Check sheet for the modelled part. Datum: model origin and axes. Units: mm. A direction names the side the tool comes from. Round coordinates to 2 decimals unless told otherwise and drop trailing zeros. Loops run counter-clockwise (first coordinate to the right, second up) from the corner with the lowest first, then second, coordinate; pieces in that order, holes last. Notation, with made-up numbers: (39.25, 15) -> (64.25, 15) arc R19 ccw to (64.25, 45) -> close; hole circle Ø5 at (62, -5). An arc over 180 degrees is marked (long way). One line per question, with ' | ' between items.
```python
from build123d import *

# Parameters (mm, degrees)
F0_W            = 116
F0_H            = 116
F1_DEPTH        = 20
F2_W            = 112
F2_H            = 112
F3_DEPTH        = 13
F4_W            = 96
F4_H            = 96
F5_DEPTH        = 7
F6_W            = 112
F6_H            = 112
F6_W_2          = 96
F6_H_2          = 96
F7_DEPTH        = 3.5
F8_W            = 10
F8_H            = 10
F9_DEPTH        = 7
F11_D           = 3.4
F11_CBORE_D     = 6.5
F11_CBORE_DEPTH = 3


with BuildPart() as f1:
    # F0 (on Top) → F1 (new body)
    with BuildSketch(Plane.XY):
        Rectangle(F0_W, F0_H)
    extrude(amount=F1_DEPTH)

    # F2 (on face) → F3 (cut)
    with BuildSketch(Plane.XY.offset(20)):
        Rectangle(F2_W, F2_H)
    extrude(amount=-F3_DEPTH, mode=Mode.SUBTRACT)

    # F4 (on face) → F5 (cut, through all)
    with BuildSketch(Plane.XY.offset(7)):
        Rectangle(F4_W, F4_H)
    extrude(amount=-F5_DEPTH, mode=Mode.SUBTRACT)

    # F6 (on face) → F7 (cut)
    with BuildSketch(Plane(origin=(0, 0, 0), x_dir=(1, 0, 0), z_dir=(0, 0, -1))):
        Rectangle(F6_W, F6_H)
        Rectangle(F6_W_2, F6_H_2, mode=Mode.SUBTRACT)
    extrude(amount=-F7_DEPTH, mode=Mode.SUBTRACT)

    # F8 (on face) → F9 (join, through all)
    with BuildSketch(Plane.XY.offset(7)):
        with Locations((-45, 45)):
            Rectangle(F8_W, F8_H)
        with Locations((45, 45)):
            Rectangle(F8_W, F8_H)
        with Locations((-45, -45)):
            Rectangle(F8_W, F8_H)
        with Locations((45, -45)):
            Rectangle(F8_W, F8_H)
    extrude(amount=-F9_DEPTH)

    # F11 (through all)
    with Locations(Plane.XY.offset(7)):
        with Locations((45, 45), (-45, 45), (-45, -45), (45, -45)):
            CounterBoreHole(F11_D / 2, F11_CBORE_D / 2, F11_CBORE_DEPTH)


solid = f1.part
```
(1) Mould release check, pull along X, two halves, no side actions. Record for faces 4 (the face through (40, 45, 4)), 5 (the face through (47, 45, 0)): +X half, -X half, draft (parallel to the pull), parting line (faces both ways), or undercut.
Answer:
face 4: undercut | face 5: draft
(2) Sectioned sample at B-B, the plane z = 11. Record the cut outline in (x, y).
Answer:
outline: (-58, -58) -> (58, -58) -> (58, 58) -> (-58, 58) -> close; hole (-56, -56) -> (56, -56) -> (56, 56) -> (-56, 56) -> close
(3) Sectioned sample at C-C, the plane y = 45. Count the separate pieces of the cut face and the enclosed holes in it, and give its area (3 significant figures).
Answer:
separate pieces: 4 | enclosed holes: 0 | area: 196 mm2
(4) Set-up check for faces 1 (the face through (46.4, 43.6, 4)), 2 (the face through (-50, -45, 2)), 3 (the face through (46.35, 43.97, 1.97)): record each of +Z, -Z, +X, -X, +Y, -Y from which the full face is reachable in a straight line by a thin tool's end or side.
Answer:
face 1: +Z | face 2: -Z | face 3: +Z, -Z
(5) Go/stop test with a flat-tipped pin: pin 1 (5 mm diameter, centred on x = 45, y = -45, fed in from +Z). Record where the tip stops, or that it passes through.
Answer:
pin 1: stops at z = 4
(6) Sectioned sample at A-A, the plane x = -33. Record the cut outline in (y, z), and give its area (3 significant figures).
Answer:
outline: (-58, 0) -> (-56, 0) -> (-56, 3.5) -> (-48, 3.5) -> (-48, 7) -> (-56, 7) -> (-56, 20) -> (-58, 20) -> close; (48, 3.5) -> (56, 3.5) -> (56, 0) -> (58, 0) -> (58, 20) -> (56, 20) -> (56, 7) -> (48, 7) -> close | area: 136 mm2
(7) Scan lines: probe 1 along Y at (x, z) = (-45, 4.75); probe 2 along Y at (x, z) = (-45, 2.8); probe 3 along Y at (x, z) = (48.5, 11). Record each from-to range of solid material in increasing order.
Answer:
probe 1: y = -58 to -48.25, -41.75 to -40, 40 to 41.75, 48.25 to 58 | probe 2: y = -58 to -56, -50 to -46.7, -43.3 to -40, 40 to 43.3, 46.7 to 50, 56 to 58 | probe 3: y = -58 to -56, 56 to 58
